For this review, take the finished solid that the model builds, in its own axes (mm). Round coordinates to 2 decimals unless told otherwise and drop trailing zeros. Order: outer loops, then holes, each group sorted by start corner. A loop starts at its lowest first (then second) coordinate and runs counter-clockwise, first axis right, second up. Notation, with made-up numbers: M 44,-27.5 L 60,-27.5 A26 ccw 60,3.5 Z; hole C 76.5,47.25 d5. An arc over 180 degrees is marked long. Put each result on its own line as item: value.
from build123d import *

# Parameters (mm, degrees)
CIRPATTERN1_COUNT = 8


with BuildPart() as part:
    # Sketch1 → Revolve2 (revolve)
    with BuildSketch(Plane.XY, mode=Mode.PRIVATE) as revolve2_sk:
        with BuildLine():
            Line((71.727523602, 109.927507641), (76.490023602, 109.927507641))
            Line((76.490023602, 109.927507641), (76.490023602, -212.127513222))
            Line((76.490023602, -212.127513222), (53.881527661, -212.127513222))
            Line((53.881527661, -212.127513222), (53.881527661, -59.727513222))
            add(Edge.make_bspline(
                [(53.881527661, -59.727513222), (53.88152643, -59.656983157), (53.880997287, -59.515406103), (53.878621437, -59.181564616), (53.872296838, -58.904795493), (53.862811351, -58.532567488), (53.850168453, -58.212837622), (53.830417626, -57.781594443), (53.800405285, -57.280959899), (53.756193121, -56.687998165), (53.677288452, -55.848480366), (53.577426861, -55.00816586), (53.456675786, -54.17243543), (53.286810822, -53.17242524), (53.092064187, -52.177442821), (52.86637512, -51.188539083), (52.610014224, -50.207489038), (52.32928934, -49.23307774), (52.024348739, -48.265969224), (51.633537831, -47.149135067), (51.139520361, -45.890408405), (50.598733753, -44.650968804), (50.012060928, -43.432701526), (49.380120231, -42.237093239), (48.704125229, -41.066154879), (47.98447552, -39.920972657), (47.223102138, -38.804076239), (46.51986906, -37.851451785), (45.893537937, -37.055672123), (45.352817681, -36.403381282), (44.915126948, -35.894247633), (44.51477619, -35.446992657), (44.181457503, -35.084631185), (43.873924624, -34.760340151), (43.674072407, -34.551549451), (43.444392073, -34.318516288), (43.343783151, -34.217162055), (43.293911001, -34.167289665)],
                knots=[0.082637729, 0.082637729, 0.082637729, 0.082637729, 0.082637729, 0.092574926, 0.102512123, 0.11244932, 0.122386517, 0.132323714, 0.142260911, 0.162135305, 0.182009699, 0.201884093, 0.24163288, 0.261507274, 0.281381668, 0.321130456, 0.360879243, 0.380753637, 0.400628031, 0.440376819, 0.480125606, 0.519874394, 0.559623181, 0.599371969, 0.639120757, 0.678869544, 0.718618332, 0.75836712, 0.798115907, 0.817990301, 0.837864695, 0.857739089, 0.877613483, 0.88755068, 0.897487877, 0.907425074, 0.91736227, 0.91736227, 0.91736227, 0.91736227, 0.91736227], degree=4))
            Line((43.293911001, -34.167289665), (34.686282803, -25.559661468))
            add(Edge.make_bspline(
                [(24.099067874, 0.000160672), (24.099069105, -0.070367974), (24.099598252, -0.213423516), (24.101973937, -0.543022243), (24.108298331, -0.823999723), (24.117783452, -1.194661398), (24.130425744, -1.513274385), (24.146225968, -1.86177893), (24.165181227, -2.193546198), (24.19281884, -2.617908727), (24.232287047, -3.121873274), (24.303299707, -3.879818002), (24.423126678, -4.886289715), (24.599486044, -6.056550088), (24.850885233, -7.385005743), (25.151795313, -8.703413843), (25.501770623, -10.009476538), (25.900360983, -11.301658927), (26.346945392, -12.577938667), (26.841003323, -13.836726817), (27.381673122, -15.076036463), (27.968479386, -16.294449129), (28.600139398, -17.489778131), (29.276532396, -18.661127095), (29.995445102, -19.805582737), (30.758021999, -20.923699417), (31.459167193, -21.874251104), (32.088736123, -22.673284825), (32.624128416, -23.320261484), (33.072255768, -23.839844364), (33.508450026, -24.329655594), (33.935826121, -24.788323739), (34.24555864, -25.11370766), (34.536859958, -25.409488397), (34.636412425, -25.509789283), (34.686282803, -25.559661468)],
                knots=[0.082637729, 0.082637729, 0.082637729, 0.082637729, 0.082637729, 0.092574926, 0.102512123, 0.11244932, 0.122386517, 0.132323714, 0.142260911, 0.152198108, 0.162135305, 0.182009699, 0.201884093, 0.24163288, 0.281381668, 0.321130456, 0.360879243, 0.400628031, 0.440376819, 0.480125606, 0.519874394, 0.559623181, 0.599371969, 0.639120757, 0.678869544, 0.718618332, 0.75836712, 0.798115907, 0.817990301, 0.837864695, 0.857739089, 0.877613483, 0.897487877, 0.907425074, 0.91736227, 0.91736227, 0.91736227, 0.91736227, 0.91736227], degree=4))
            add(Edge.make_bspline(
                [(24.099067874, 0.000160672), (24.0990685, 0.036053324), (24.099606331, 0.110274362), (24.102023723, 0.267801742), (24.108461568, 0.427224789), (24.120533599, 0.646924939), (24.141435087, 0.901594), (24.175184719, 1.202697945), (24.226499305, 1.54221117), (24.290543701, 1.881157449), (24.367141601, 2.216515092), (24.456323571, 2.549400093), (24.557741413, 2.878253317), (24.671619071, 3.203507713), (24.797196771, 3.523787829), (24.935285977, 3.839827405), (25.084070301, 4.149442857), (25.246012222, 4.454943795), (25.416488505, 4.751462248), (25.602514721, 5.045864533), (25.79178827, 5.325679608), (26.004405474, 5.610888215), (26.178876374, 5.83307432), (26.366345756, 6.050112309), (26.504555248, 6.208802318), (26.67044207, 6.382282451), (26.744520261, 6.458639514), (26.795279203, 6.509400323)],
                knots=[0.082568816, 0.082568816, 0.082568816, 0.082568816, 0.082568816, 0.102426634, 0.122284453, 0.142142271, 0.162000089, 0.201715725, 0.241431362, 0.281146998, 0.320862634, 0.360578271, 0.400293907, 0.440009544, 0.47972518, 0.519440816, 0.559156453, 0.598872089, 0.638587725, 0.678303362, 0.718018998, 0.757734635, 0.797450271, 0.837165907, 0.857023726, 0.876881544, 0.91659718, 0.91659718, 0.91659718, 0.91659718, 0.91659718], degree=4))
            add(Edge.make_bspline(
                [(26.795279203, 6.509400323), (49.261401403, 34.636114842), (71.727523602, 109.927507641)],
                knots=[0, 0, 0, 1, 1, 1], degree=2))
        make_face()
    revolve(revolve2_sk.sketch.rotate(Axis((-0.005532126, 165.815985114, 0), (0, -1, 0)), 180), axis=Axis((-0.005532126, 165.815985114, 0), (0, -1, 0)))

    # Sketch4 → 3/8-24 Tapped Hole1 (revolve, cut)
    with BuildSketch(Plane(origin=(65.2, -212.127513222, 0), x_dir=(0, 0, -1), z_dir=(1, 0, 0))):
        Polygon((0, 0), (0, 27.533468714), (4.2164, 25), (4.2164, 0), align=None)
    f_3_8_24_tapped_hole1 = revolve(axis=Axis((65.2, -218.477513222, 0), (0, 1, 0)), mode=Mode.SUBTRACT)

    # CirPattern1: 3/8-24 Tapped Hole1 ×8 about axis
    cirpattern1_axis = Axis((0, -228.487022387, 0), (-1.634718801334702e-05, 0.9999999998663848, 0))
    for i in range(1, CIRPATTERN1_COUNT):
        add(f_3_8_24_tapped_hole1.rotate(cirpattern1_axis, i * 360 / CIRPATTERN1_COUNT), mode=Mode.SUBTRACT)


solid = part.part
(1) Insertion check: pin 1 Ø6.5 at (x, z) = (65.2, 0) entering from -Y; pin 2 Ø11 at (x, z) = (-46.1, 46.1) entering from -Y; pin 3 Ø4 at (x, y) = (-21.5, 27) entering from -Z; pin 4 Ø1.5 at (y, z) = (-70.5, -37.5) entering from +X. Each pin has a flat end and moves straight along its axis. Give the tip position at first contact, or say it passes through.
A:
pin 1: stops at y = -186.55
pin 2: stops at y = -212.13
pin 3: stops at z = -73.97
pin 4: stops at x = 67.08
(2) Add section A-A on y = -156. Give the boundary of the cut face in (x, z).
A:
outline: C -0.01,0 d152.99; hole C -0.01,0 d107.77
(3) To check wall thickness, follow L1, parallel to Z at x = -25, y = 81; L2, parallel to X at y = -181.5, z = 5; L3, parallel to Z at x = 27.5, y = -98.5. State the ranges of each line that lie inside material, in increasing order.
A:
L1: z = -72.3 to -57.29, 57.29 to 72.3
L2: x = -76.34 to -53.66, 53.65 to 76.33
L3: z = -71.38 to -46.34, 46.34 to 71.38
(4) Draft analysis for pull direction X (two halves, no side actions). For faces 1 (the face through (9.953, -53.354, -75.845)), 2 (the face through (-41.99, -199.8, 45.19)), 3 (the face through (51.3, -212.128, -17.4)), state which applies: released by +X, released by -X, zero draft, split by the parting line, or undercut.
A:
face 1: split by the parting line
face 2: undercut
face 3: zero draft
